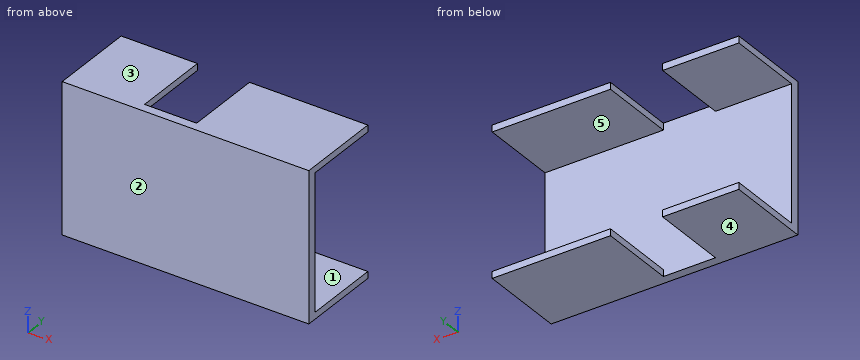
```python
from build123d import *

# Parameters (mm, degrees)
EXTRUDE_1_DEPTH = 4
SKETCH_1_3_W    = 52.77
SKETCH_1_3_H    = 3
SKETCH_1_3_W_2  = 34
EXTRUDE_2_DEPTH = 38.5


with BuildPart() as part:
    # Sketch 1 → Extrude 1 (new body)
    with BuildSketch(Plane(origin=(0, 0, 0), x_dir=(1, 0, 0), z_dir=(0, 1, 0))):
        Polygon((0, 63.5), (0, 3), (34, 3), (34, 0), (57.23, 0), (57.23, 3), (110, 3), (110, 63.5), (57.23, 63.5), (57.23, 66.5), (34, 66.5), (34, 63.5), align=None)
    extrude(amount=EXTRUDE_1_DEPTH)

    # Sketch 1_3 → Extrude 2 (add)
    with BuildSketch(Plane(origin=(0, 0, 0), x_dir=(1, 0, 0), z_dir=(0, 1, 0))):
        with Locations((83.615, 65)):
            Rectangle(SKETCH_1_3_W, SKETCH_1_3_H)
        with Locations((17, 65)):
            Rectangle(SKETCH_1_3_W_2, SKETCH_1_3_H)
        with Locations((17, 1.5)):
            Rectangle(SKETCH_1_3_W_2, SKETCH_1_3_H)
        with Locations((83.615, 1.5)):
            Rectangle(SKETCH_1_3_W, SKETCH_1_3_H)
    extrude(amount=EXTRUDE_2_DEPTH)


solid = part.part
```
The listing builds one solid part. Answer for the finished solid, in the listing's coordinates (mm). Face numbers are marked on the shaded views. A direction names the side the tool comes from. Coordinates: 2 decimals unless noted, no trailing zeros. Write each loop counter-clockwise with the first axis right and the second up, starting at its lowest first coordinate (ties: lowest second). Pieces come first, ordered by that corner, then holes. Notation, with made-up numbers: (33.5, -20) - (56.5, -20) arc R8 ccw to (56.5, -7) - close; hole circle Ø6 at (-20.5, 50.25). An arc over 180 degrees is marked (long way). Return JSON: item names as keys, results as strings. Group by question number.
Q1. Which of the six approach directions +Z, -Z, +X, -X, +Y, -Y give full straight-line access (tool end or side, diameter ignored) to the marked faces 4 and 5?
Q2. The part is cut by section C-C on z = -5. Write down the section's boundary in (x, y), and give its area (3 significant figures).
Q3. The part is cut by section A-A on y = 35.5. Write down the section's boundary in (x, z), and give its area (3 significant figures).
Q4. Find the intervals of material crossed by line 1 along Z through (x, y) = (72, 29); line 2 along Y through (x, z) = (28.5, -49), in increasing order. Write a range as [from, to].
Q5. The part is cut by section D-D on x = 47. Write down the section's boundary in (y, z), and give its area (3 significant figures).
Q6. The part is cut by section B-B on x = 14.5. Write down the section's boundary in (y, z).
Q7. Flat-ended cylindrical pins translate along their axes: pin 1 Ø6 at (x, y) = (17.5, 26.5) entering from +Z; pin 2 Ø20 at (x, z) = (56, -36.5) entering from +Y. Find the tip coordinate at first contact, or state that the pin passes through.
Q8. For a pull along Z with two mould halves and no side action, classify the marked faces 1, 2 and 3 as +Z half, -Z half, draft (parallel to the pull), parting line (faces both ways), or undercut.
Evaluation:
{
 "1": {"face 4": "-Z, +X, -X, +Y, -Y", "face 5": "+X, -X, +Y"},
 "2": {"outline": "(0, 0) - (110, 0) - (110, 4) - (0, 4) - close", "area": "440 mm2"},
 "3": {"outline": "(0, -66.5) - (34, -66.5) - (34, -63.5) - (0, -63.5) - close; (0, -3) - (34, -3) - (34, 0) - (0, 0) - close; (57.23, -66.5) - (110, -66.5) - (110, -63.5) - (57.23, -63.5) - close; (57.23, -3) - (110, -3) - (110, 0) - (57.23, 0) - close", "area": "521 mm2"},
 "4": {"line 1": "z = [-66.5, -63.5], [-3, 0]", "line 2": "y = [0, 4]"},
 "5": {"outline": "(0, -66.5) - (4, -66.5) - (4, 0) - (0, 0) - close", "area": "266 mm2"},
 "6": {"outline": "(0, -66.5) - (38.5, -66.5) - (38.5, -63.5) - (4, -63.5) - (4, -3) - (38.5, -3) - (38.5, 0) - (0, 0) - close"},
 "7": {"pin 1": "stops at z = 0", "pin 2": "stops at y = 4"},
 "8": {"face 1": "undercut", "face 2": "draft", "face 3": "+Z half"}
}
